Verification items for the finished model (mm, model axes). Give positions to 0.01 mm unless a question says otherwise; leave off trailing zeros. Order: outer loops, then holes, each group sorted by start corner. A loop starts at its lowest first (then second) coordinate and runs counter-clockwise, first axis right, second up.
from build123d import *

# Parameters (mm, degrees)
SKETCH1_W           = 249.6
SKETCH1_H           = 150
BOSS_EXTRUDE1_DEPTH = 3
SKETCH2_R           = 20
CUT_EXTRUDE1_DEPTH  = 4
SKETCH3_W           = 40
SKETCH3_H           = 30
CUT_EXTRUDE2_DEPTH  = 5
SKETCH4_R           = 2.1
SKETCH4_R_2         = 4
CUT_EXTRUDE3_DEPTH  = 4


with BuildPart() as part:
    # Sketch1 → Boss-Extrude1 (new body)
    with BuildSketch(Plane.XY):
        with Locations((124.8, -75)):
            Rectangle(SKETCH1_W, SKETCH1_H)
    extrude(amount=BOSS_EXTRUDE1_DEPTH)

    # Sketch2 → Cut-Extrude1 (cut, through all)
    with BuildSketch(Plane.XY.offset(3)):
        with Locations((67.5, -69.58494332)):
            Circle(SKETCH2_R)
    extrude(amount=-CUT_EXTRUDE1_DEPTH, mode=Mode.SUBTRACT)

    # Sketch3 → Cut-Extrude2 (cut)
    with BuildSketch(Plane.XY.offset(3)):
        with Locations((229.6, -104.652337216)):
            Rectangle(SKETCH3_W, SKETCH3_H)
    extrude(amount=-CUT_EXTRUDE2_DEPTH, mode=Mode.SUBTRACT)

    # Sketch4 → Cut-Extrude3 (cut, through all)
    with BuildSketch(Plane.XY.offset(3)):
        with Locations((244.6, -120.152337216)):
            Circle(SKETCH4_R)
        with Locations((227.1, -120.152337216)):
            Circle(SKETCH4_R)
        with Locations((239.6, -107.652337216)):
            Circle(SKETCH4_R_2)
        with Locations((244.6, -95.152337216)):
            Circle(SKETCH4_R)
        with Locations((227.1, -95.152337216)):
            Circle(SKETCH4_R)
        with Locations((202.1, -120.152337216)):
            Circle(SKETCH4_R)
        with Locations((202.1, -95.152337216)):
            Circle(SKETCH4_R)
        with Locations((214.6, -107.652337216)):
            Circle(SKETCH4_R_2)
    extrude(amount=-CUT_EXTRUDE3_DEPTH, mode=Mode.SUBTRACT)


solid = part.part
(1) Section check A-A, the plane x = 67.5. Enter the section's corners in (y, z), then the cut area to 3 significant figures.
Solved:
outline: (-150, 0) - (-89.58, 0) - (-89.58, 3) - (-150, 3) - close; (-49.58, 0) - (0, 0) - (0, 3) - (-49.58, 3) - close
area: 330 mm2
(2) Scan lines: line 1 (Y direction, x = 202.1, z = 0.8); line 2 (Y direction, x = 216.5, z = 1.9); line 3 (Y direction, x = 203, z = 2). Record each from-to range of solid material in increasing order.
Solved:
line 1: y = -150 to -122.25, -118.05 to -97.25, -93.05 to 0
line 2: y = -150 to -119.65, -89.65 to 0
line 3: y = -150 to -122.05, -118.25 to -97.05, -93.25 to 0
(3) Release check for a two-part mould opening along X. For faces 1 (the flat face through (123, -74, 0)), 2 (the cylindrical face through (76.73, -87.33, 1.52)) record: pulls with the +X half, pulls with the -X half, needs draft (parallel to the pull), parting line crosses it, or undercut.
Solved:
face 1: needs draft
face 2: undercut
(4) Go/stop test with a flat-tipped pin: pin 1 (10 mm diameter, centred on x = 76, y = -87, fed in from -Z). Record where the tip stops, or that it passes through.
Solved:
pin 1: stops at z = 0
(5) Section check C-C, the plane z = 2.15. Enter the section's corners in (x, y), then the cut area to 3 significant figures.
Solved:
outline: (0, -150) - (249.6, -150) - (249.6, -119.65) - (246.64, -119.65) arc R2.1 cw (long way) to (242.56, -119.65) - (229.14, -119.65) arc R2.1 cw (long way) to (225.06, -119.65) - (209.6, -119.65) - (209.6, -89.65) - (249.6, -89.65) - (249.6, 0) - (0, 0) - close; hole circle Ø40 at (67.5, -69.58); hole circle Ø4.2 at (202.1, -120.15); hole circle Ø4.2 at (202.1, -95.15)
area: 34,900 mm2
(6) Section check B-B, the plane y = -64. Enter the section's corners in (x, z), then the cut area to 3 significant figures.
Solved:
outline: (0, 0) - (48.3, 0) - (48.3, 3) - (0, 3) - close; (86.7, 0) - (249.6, 0) - (249.6, 3) - (86.7, 3) - close
area: 634 mm2
